Answer from the drawing. Dimensions are ordinates in mm from the lowest x, y and z of the part. A direction names the side the tool comes from. Round coordinates to 2 decimals unless told otherwise and drop trailing zeros. Order: outer loops, then holes, each group sorted by start corner. A loop starts at its lowest first (then second) coordinate and runs counter-clockwise, first axis right, second up. Notation, with made-up numbers: (-11, 10) -> (8, 10) arc R26 cw to (8, 30) -> close; hole circle Ø7 at (11.5, 1.5). An arc over 180 degrees is marked (long way). Use a Markdown table: item, result. Add a question column.
1. The mould has two halves that part along Z. Classify the marked faces 1, 2 and 3: +Z half, -Z half, draft (parallel to the pull), parting line (faces both ways), or undercut.
2. Section D-D, the plane z = 20.5 is taken. Give the vertices of the cut face in (x, y) (1 decimal).
3. Section A-A, the plane x = 45 is taken. Give the vertices of the cut face in (y, z).
4. Given pin 1 (4 mm diameter, centred on y = 7, z = 40, fed in from +X), flat-ended and moving along its own axis, determine where the tip first touches the part or whether it passes through.
5. Section B-B, the plane z = 13 is taken. Give the vertices of the cut face in (x, y), then the cut area to 3 significant figures.
6. For the marked faces 4 and 5, determine the directions among +Z, -Z, +X, -X, +Y, -Y from which every point of the face is accessible in a straight line to the end or side of a thin tool.
7. Consider L1, parallel to X at y = 8.5, z = 17 (1 decimal); L2, parallel to Z at x = 34, y = 8 (1 decimal); L3, parallel to X at y = 9, z = 20 (1 decimal). Determine where each line is inside the solid, lowest interval first. Write a range as [from, to].
8. Section C-C, the plane y = 4.25 is taken. Give the number of separate pieces and of enclosed holes in the cut face, then the cut area to 4 significant figures.
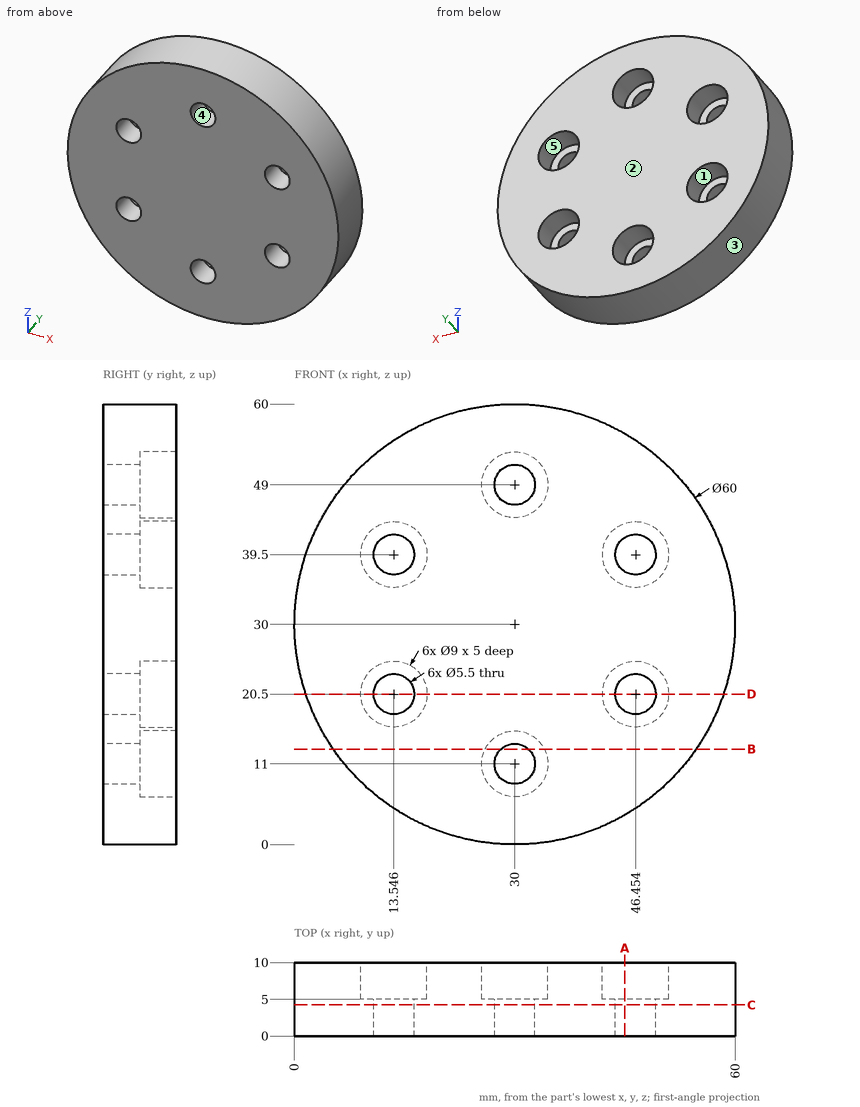
Verdict:
| question | item | result |
|---|---|---|
| 1 | face 1 | undercut |
| 1 | face 2 | draft |
| 1 | face 3 | parting line |
| 2 | outline | (1.5, 0) -> (10.8, 0) -> (10.8, 5) -> (9, 5) -> (9, 10) -> (1.5, 10) -> close; (16.3, 0) -> (43.7, 0) -> (43.7, 5) -> (42, 5) -> (42, 10) -> (18, 10) -> (18, 5) -> (16.3, 5) -> close; (49.2, 0) -> (58.5, 0) -> (58.5, 10) -> (51, 10) -> (51, 5) -> (49.2, 5) -> close |
| 3 | outline | (0, 4.02) -> (10, 4.02) -> (10, 16.24) -> (5, 16.24) -> (5, 18.17) -> (0, 18.17) -> close; (0, 22.83) -> (5, 22.83) -> (5, 24.76) -> (10, 24.76) -> (10, 35.24) -> (5, 35.24) -> (5, 37.17) -> (0, 37.17) -> close; (0, 41.83) -> (5, 41.83) -> (5, 43.76) -> (10, 43.76) -> (10, 55.98) -> (0, 55.98) -> close |
| 4 | pin 1 | stops at x = 58.91 |
| 5 | outline | (5.28, 0) -> (28.11, 0) -> (28.11, 5) -> (25.97, 5) -> (25.97, 10) -> (5.28, 10) -> close; (31.89, 0) -> (54.72, 0) -> (54.72, 10) -> (34.03, 10) -> (34.03, 5) -> (31.89, 5) -> close |
| 5 | area | 435 mm2 |
| 6 | face 4 | +Y, -Y |
| 6 | face 5 | +Y |
| 7 | L1 | x = [3, 10.7], [16.4, 43.6], [49.3, 57] |
| 7 | L2 | z = [0.3, 8.9], [13.1, 46.9], [51.1, 59.7] |
| 7 | L3 | x = [1.7, 9.1], [18, 42], [50.9, 58.3] |
| 8 | separate pieces | 1 |
| 8 | enclosed holes | 6 |
| 8 | area | 2,685 mm2 |
